```python
from build123d import *

# Parameters (mm, degrees)
F0_W      = 254
F0_H      = 254
F1_DEPTH  = 508
F2_SIZE   = 127
F3_SIZE   = 126.99999
F4_W      = 110.2521903813
F4_H      = 222.1985608339
F5_DEPTH  = 12.7
F6_R      = 15.2445630658
F7_DEPTH  = 25.4
F8_W      = 60.8862751365
F8_H      = 17.78
F9_DEPTH  = 12.7
F10_W     = 44.4203019142
F10_H     = 51.6851246357
F10_W_2   = 47.3152212799
F10_H_2   = 46.0566580296
F10_W_3   = 41.5758583695
F10_H_3   = 51.8873212337
F10_W_4   = 40.2868166566
F10_H_4   = 50.077855587
F11_DEPTH = 25.4
F12_W     = 67.7322521806
F12_H     = 71.3757276535
F13_DEPTH = 127
F14_W     = 210.3085294366
F14_H     = 119.9935823679
F15_DEPTH = 228.6
F16_W     = 37.6376099885
F16_H     = 126.9762441516
F16_W_2   = 43.185967952
F16_H_2   = 134.4709768891
F16_W_3   = 35.2269485593
F16_H_3   = 143.0262625217
F17_DEPTH = 25.4
F18_R     = 26.1262901257
F18_R_2   = 20.0737439282
F18_R_3   = 29.9342227193
F19_DEPTH = 12.7
F20_W     = 29.2137209326
F20_H     = 63.1077764034
F20_H_2   = 23.1252685189
F20_W_2   = 94.6274452358
F20_W_3   = 130.1588338315
F20_H_3   = 76.8547430634
F21_DEPTH = 25.4


# Not quite as in the source:
# - a fillet or chamfer is up to 0.001 mm smaller than in the source, because OpenCascade refuses the exact size


with BuildPart() as f1:
    # F0 (on Top) → F1 (new body)
    with BuildSketch(Plane.XY):
        with Locations((3.1588338315, -4.6172558538)):
            Rectangle(F0_W, F0_H)
    extrude(amount=F1_DEPTH)

    # F2
    f2_edges = [f1.edges().sort_by_distance(p)[0] for p in [
        (3.158834, -131.617256, 508),
    ]]
    chamfer(f2_edges, length=F2_SIZE)

    # F3 (size 127 in the source; OpenCascade refuses exactly that, so slightly less here)
    f3_edges = [f1.edges().sort_by_distance(p)[0] for p in [
        (3.158834, 122.382744, 508),
    ]]
    chamfer(f3_edges, length=F3_SIZE)

    # F4 (on face) → F5 (join)
    with BuildSketch(Plane(origin=(-123.8411661685, 0, 0), x_dir=(0, -1, 0), z_dir=(-1, 0, 0))):
        with Locations((3.7376638502, 111.099280417)):
            Rectangle(F4_W, F4_H)
    extrude(amount=F5_DEPTH)

    # F6 (on face) → F7 (join)
    with BuildSketch(Plane(origin=(-136.5411661685, 0, 0), x_dir=(0, -1, 0), z_dir=(-1, 0, 0))):
        with Locations((41.2117242813, 101.0684147477)):
            Circle(F6_R)
    extrude(amount=F7_DEPTH)

    # F8 (on face) → F9 (join)
    with BuildSketch(Plane(origin=(-161.9411661685, 0, 0), x_dir=(0, -1, 0), z_dir=(-1, 0, 0))):
        with Locations((22.795823104, 100.5913294025)):
            Rectangle(F8_W, F8_H)
    extrude(amount=F9_DEPTH)

    # F10 (on face) → F11 (cut)
    with BuildSketch(Plane(origin=(-123.8411661685, 0, 0), x_dir=(0, -1, 0), z_dir=(-1, 0, 0))):
        with Locations((-22.2101509571, 357.1109622717)):
            Rectangle(F10_W, F10_H)
        with Locations((-23.6576106399, 284.112855792)):
            Rectangle(F10_W_2, F10_H_2)
        with Locations((38.0553556606, 355.0563393831)):
            Rectangle(F10_W_3, F10_H_3)
        with Locations((38.7203507125, 285.8152091503)):
            Rectangle(F10_W_4, F10_H_4)
    extrude(amount=-F11_DEPTH, mode=Mode.SUBTRACT)

    # F12 (on face) → F13 (join)
    with BuildSketch(Plane(origin=(0, 251.6913720731, 251.6913720731), x_dir=(-1, 0, 0), z_dir=(0, 0.7071067812, 0.7071067812))):
        with Locations((-33.8661260903, 287.2642278671)):
            Rectangle(F12_W, F12_H)
    extrude(amount=F13_DEPTH)

    # F14 (on face) → F15 (cut)
    with BuildSketch(Plane.XZ.offset(131.6172558538)):
        with Locations((-3.9455778897, 294.7669550776)):
            Rectangle(F14_W, F14_H)
    extrude(amount=-F15_DEPTH, mode=Mode.SUBTRACT)

    # F16 (on face) → F17 (join)
    with BuildSketch(Plane.XY.offset(234.7701638937)):
        with Locations((-53.3800702542, -6.8131200969)):
            Rectangle(F16_W, F16_H)
        with Locations((4.870776087, -3.0657537282)):
            Rectangle(F16_W_2, F16_H_2)
        with Locations((68.4281103313, 1.2118890882)):
            Rectangle(F16_W_3, F16_H_3)
    extrude(amount=F17_DEPTH)

    # F18 (on face) → F19 (join)
    with BuildSketch(Plane.XY.offset(260.1701638937)):
        with Locations((-53.3800702542, 75.6483599544)):
            Circle(F18_R)
        with Locations((0, 86.5157917142)):
            Circle(F18_R_2)
        with Locations((55.7353012264, 86.5157917142)):
            Circle(F18_R_3)
    extrude(amount=F19_DEPTH)

    # F20 (on face) → F21 (join)
    with BuildSketch(Plane.XZ.offset(131.6172558538)):
        with Locations((-14.6068604663, 349.4461117983)):
            Rectangle(F20_W, F20_H)
        with Locations((-14.6068604663, 306.3295893371)):
            Rectangle(F20_W, F20_H_2)
        with Locations((-76.5274435505, 306.3295893371)):
            Rectangle(F20_W_2, F20_H_2)
        with Locations((65.0794169158, 306.3295893371)):
            Rectangle(F20_W_3, F20_H_2)
        with Locations((-14.6068604663, 256.3395835459)):
            Rectangle(F20_W, F20_H_3)
    extrude(amount=-F21_DEPTH)


solid = f1.part
```
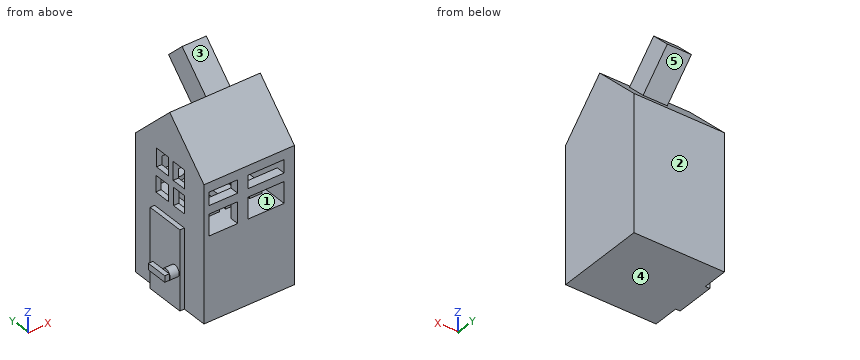
Input: part model. Units: mm. Frame: model coordinates. Face numbers are marked on the shaded views. A direction names the side the tool comes from. Give positions to 0.01 mm unless a question says otherwise; leave off trailing zeros. Loops run counter-clockwise (first coordinate to the right, second up) from the corner with the lowest first, then second, coordinate; pieces in that order, holes last. Notation, with made-up numbers: (19.5, -9.75) -> (77.5, -9.75) arc R38 ccw to (77.5, 29.25) -> close; hole circle Ø5 at (-17, 74.25). An arc over 180 degrees is marked (long way). Use a Markdown table: item, result.
Q1. First-contact query: P1, Ø13, axis at y = -35, z = 368.5, coming from the -X side; P2, Ø12, axis at x = -51, z = 321.5, coming from the +Y side; P3, Ø7.5, axis at y = -124, z = 269.5, coming from the -X side. Flat tips, straight axial feed; report the tip coordinate or a pass-through.
Entries:
| item | result |
|---|---|
| P1 | stops at x = -98.44 |
| P2 | stops at y = 122.38 |
| P3 | stops at x = -123.84 |
Q2. Access query for the marked faces 4 and 5. Directions: +Z, -Z, +X, -X, +Y, -Y. A direction counts if a zero-diameter tool reaches every point of the face in a straight line with its end or side. Return the directions, or none.
Entries:
| item | result |
|---|---|
| face 4 | -Z, +X, -X, +Y, -Y |
| face 5 | +X, -X, +Y |
Q3. Pull-direction query (Z, two-part tool) for the marked faces 1, 2 and 3; classes: pulls with the +Z half, pulls with the -Z half, needs draft (parallel to the pull), parting line crosses it, or undercut.
Entries:
| item | result |
|---|---|
| face 1 | undercut |
| face 2 | needs draft |
| face 3 | pulls with the +Z half |
Q4. Section query A-A, the plane z = 52.5. Return the cut outline in (x, y), plus the area to 3 significant figures.
Entries:
| item | result |
|---|---|
| outline | (-136.54, -58.86) -> (-123.84, -58.86) -> (-123.84, -131.62) -> (130.16, -131.62) -> (130.16, 122.38) -> (-123.84, 122.38) -> (-123.84, 51.39) -> (-136.54, 51.39) -> close |
| area | 65,900 mm² |
Q5. Section query D-D, the plane x = -151. Return the cut outline in (y, z).
Entries:
| item | result |
|---|---|
| outline | circle Ø30.49 at (-41.21, 101.07) |
Q6. Section query C-C, the plane z = 491.5. Return the cut outline in (x, y), plus the area to 3 significant figures.
Entries:
| item | result |
|---|---|
| outline | (-123.84, -21.12) -> (130.16, -21.12) -> (130.16, 11.88) -> (-123.84, 11.88) -> close; (0, 34.78) -> (67.73, 34.78) -> (67.73, 135.72) -> (0, 135.72) -> close |
| area | 15,200 mm² |
Q7. Ray query, probe 1 along Y at (x, z) = (-15.5, 245); probe 2 along X at (y, z) = (-15, 103); probe 3 along Y at (x, z) = (-70.5, 155). Return the intervals inside material, ascending. Write a range as from..to.
Entries:
| item | result |
|---|---|
| probe 1 | y = -131.62..-106.22, -70.3..64.17, 96.98..122.38 |
| probe 2 | x = -174.64..-161.94, -136.54..130.16 |
| probe 3 | y = -131.62..122.38 |
